from build123d import *

# Parameters (mm, degrees)
F0_W     = 18
F0_H     = 20
F0_W_2   = 42
F1_DEPTH = 17
F2_T     = -1.5


with BuildPart() as f1:
    # F0 (on Front) → F1 (new body)
    with BuildSketch(Plane.XZ):
        with Locations((9, 10)):
            Rectangle(F0_W, F0_H)
        Polygon((18, 0), (0, 0), (18, -7), align=None)
        with Locations((39, 10)):
            Rectangle(F0_W_2, F0_H)
        Polygon((60, 0), (18, 0), (18, -7), align=None)
        Polygon((18, 27), (0, 20), (18, 20), align=None)
        Polygon((18, 27), (18, 20), (60, 20), align=None)
    extrude(amount=F1_DEPTH)

    # F2
    f2_openings = [f1.faces().sort_by_distance(p)[0] for p in [
        (28.962963, -17, 10),
    ]]
    offset(amount=F2_T, openings=f2_openings)


solid = f1.part
Geometry check sheet. Reference: the model listing, model coordinates, mm. A direction names the side the tool comes from. Coordinates: 2 decimals unless noted, no trailing zeros. Order: outer loops, then holes, each group sorted by start corner. A loop starts at its lowest first (then second) coordinate and runs counter-clockwise, first axis right, second up. Notation, with made-up numbers: (-9.75, 63.5) - (49.25, 63.5) arc R25 ccw to (49.25, 94.5) - close; hole circle Ø1 at (45.25, 52.25). An arc over 180 degrees is marked (long way). Answer in a Markdown table with one row per item. Add a question column.
1) Cross-section at C-C, the plane z = 9.5. Record the cut outline in (x, y), then the cut area to 4 significant figures.
2) Cross-section at B-B, the plane x = 34. Record the cut outline in (y, z), then the cut area to 3 significant figures.
3) Cross-section at A-A, the plane y = -9. Record the cut outline in (x, z).
4) Release check for a two-part mould opening along Z. For faces 1 (the flat face through (30, 0, 10)), 2 (the flat face through (9.95, -9.14, 22.26)), 3 (the flat face through (39.29, -8.38, 23.45)) record: +Z half, -Z half, draft (parallel to the pull), parting line (faces both ways), or undercut.
5) Material ranges on line 1 along X through (y, z) = (-3.5, 14); line 2 along Y through (x, z) = (6.5, 20); line 3 along Z through (x, y) = (49, -11.5), recorded low to high. Write a range as [from, to].
6) Set-up check for faces 4 (the flat face through (8.87, -8.38, -3.45)), 5 (the flat face through (58.5, -9, 10)): record each of +Z, -Z, +X, -X, +Y, -Y from which the full face is reachable in a straight line by a thin tool's end or side.
7) Gauge pin test, flat ends, axial feed: P1, Ø4, axis at x = 48, y = -7.5, coming from the -Z side; P2, Ø6, axis at x = 30, z = 12, coming from the -Y side; P3, Ø5, axis at x = 37.5, y = -13.5, coming from the +Z side. Record the tip position at first contact, or that the pin passes through.
Check result:
| question | item | result |
|---|---|---|
| 1 | outline | (0, -17) - (1.5, -17) - (1.5, -1.5) - (58.5, -1.5) - (58.5, -17) - (60, -17) - (60, 0) - (0, 0) - close |
| 1 | area | 136.5 mm² |
| 2 | outline | (-17, -4.33) - (0, -4.33) - (0, 24.33) - (-17, 24.33) - (-17, 22.81) - (-1.5, 22.81) - (-1.5, -2.81) - (-17, -2.81) - close |
| 2 | area | 90.1 mm² |
| 3 | outline | (0, 0) - (18, -7) - (60, 0) - (60, 20) - (18, 27) - (0, 20) - close; hole (1.5, 1.03) - (18.16, -5.45) - (58.5, 1.27) - (58.5, 18.73) - (18.16, 25.45) - (1.5, 18.97) - close |
| 4 | face 1 | draft |
| 4 | face 2 | undercut |
| 4 | face 3 | +Z half |
| 5 | line 1 | x = [0, 1.5], [58.5, 60] |
| 5 | line 2 | y = [-1.5, 0] |
| 5 | line 3 | z = [-1.83, -0.31], [20.31, 21.83] |
| 6 | face 4 | -Z, -X, +Y, -Y |
| 6 | face 5 | -Y |
| 7 | P1 | stops at z = -2.33 |
| 7 | P2 | stops at y = -1.5 |
| 7 | P3 | stops at z = 24.17 |
